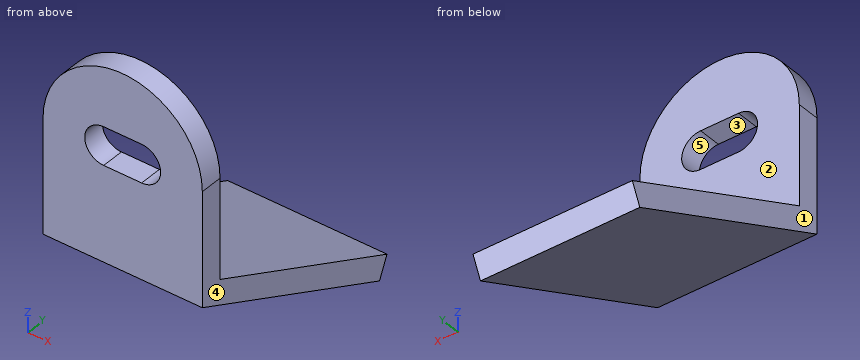
from build123d import *

# Parameters (mm, degrees)
BOSS_EXTRUDE1_DEPTH = 3
BOSS_EXTRUDE3_DEPTH = 21


with BuildPart() as part:
    # Sketch1 → Boss-Extrude1 (new body)
    with BuildSketch(Plane(origin=(0, 0, 0), x_dir=(1, 0, 0), z_dir=(0, 1, 0))):
        with BuildLine():
            Line((-10.5, 0), (-10.5, 15))
            Line((-10.5, 15), (10.5, 15))
            Line((10.5, 15), (10.5, 0))
            ThreePointArc((10.5, 0), (0, -10.5), (-10.5, 0))
        make_face()
        with BuildLine():
            Line((-2.5, 2.5), (2.5, 2.5))
            ThreePointArc((2.5, 2.5), (5, 0), (2.5, -2.5))
            Line((2.5, -2.5), (-2.5, -2.5))
            ThreePointArc((-2.5, -2.5), (-5, 0), (-2.5, 2.5))
        make_face(mode=Mode.SUBTRACT)
    extrude(amount=BOSS_EXTRUDE1_DEPTH)

    # Sketch3 → Boss-Extrude3 (add)
    with BuildSketch(Plane(origin=(10.5, 0, 0), x_dir=(0, 0, -1), z_dir=(1, 0, 0))):
        Polygon((15, 0), (28.989229745, 30), (26.270306384, 31.267854785), (11.689866243, 0), align=None)
    extrude(amount=-BOSS_EXTRUDE3_DEPTH)


solid = part.part
Input: part model. Units: mm. Frame: model coordinates. Face numbers are marked on the shaded views. A direction names the side the tool comes from. Coordinates: 2 decimals unless noted, no trailing zeros. Loops run counter-clockwise (first coordinate to the right, second up) from the corner with the lowest first, then second, coordinate; pieces in that order, holes last. Notation, with made-up numbers: (-21, 48.5) - (14, 48.5) arc R18 ccw to (14, 67.5) - close; hole circle Ø8 at (36, -30.5). An arc over 180 degrees is marked (long way). Answer in a Markdown table with one row per item. Add a question column.
Item 1: Section query B-B on z = -2. Return the cut outline in (x, y).
Item 2: Access query for the marked faces 4 and 5. Directions: +Z, -Z, +X, -X, +Y, -Y. A direction counts if a zero-diameter tool reaches every point of the face in a straight line with its end or side. Return the directions, or none.
Item 3: Contact query for flat-ended pins moving along their axis: P1, Ø2, axis at x = -5, y = 23, coming from the -Z side; P2, Ø1, axis at x = -2, y = 5.5, coming from the -Z side; P3, Ø8, axis at x = 7, y = 24.5, coming from the -Z side. Output: stop coordinate, or through.
Item 4: Section query C-C on x = -4.5. Return the cut outline in (y, z).
Item 5: Mould query, pull axis X, two halves, no side actions, for the marked faces 1, 2 and 3. Classes: released by +X, released by -X, zero draft, split by the parting line, or undercut.
Item 6: Line query: line 1 along Y through (x, z) = (5.75, 6); line 2 along Y through (x, z) = (6.75, -24); line 3 along Z through (x, y) = (9, 15.5). Output: solid intervals per line, ascending. Write a range as [from, to].
Item 7: Section query A-A on x = 0. Return the cut outline in (y, z).
Item 8: Section query D-D on z = -10. Return the cut outline in (x, y), then the cut area to 3 significant figures.
Recorded:
| question | item | result |
|---|---|---|
| 1 | outline | (-10.5, 0) - (-4, 0) - (-4, 3) - (-10.5, 3) - close; (4, 0) - (10.5, 0) - (10.5, 3) - (4, 3) - close |
| 2 | face 4 | +Z, -Z, +X, +Y, -Y |
| 2 | face 5 | +Y, -Y |
| 3 | P1 | z = -26.19 |
| 3 | P2 | z = -17.8 |
| 3 | P3 | z = -28.29 |
| 4 | outline | (0, -15) - (30, -28.99) - (31.27, -26.27) - (3, -13.09) - (3, -1.5) - (0, -1.5) - close; (0, 1.5) - (3, 1.5) - (3, 9.49) - (0, 9.49) - close |
| 5 | face 1 | released by -X |
| 5 | face 2 | zero draft |
| 5 | face 3 | undercut |
| 6 | line 1 | [0, 3] |
| 6 | line 2 | [19.3, 26.4] |
| 6 | line 3 | [-22.23, -18.92] |
| 7 | outline | (0, -15) - (30, -28.99) - (31.27, -26.27) - (3, -13.09) - (3, -2.5) - (0, -2.5) - close; (0, 2.5) - (3, 2.5) - (3, 10.5) - (0, 10.5) - close |
| 8 | outline | (-10.5, 0) - (10.5, 0) - (10.5, 3) - (-10.5, 3) - close |
| 8 | area | 63.0 mm^2 |
